Geometry: see drawing. Coordinates: mm, zero at the bounding-box minimum. Coordinates: 2 decimals unless noted, no trailing zeros. Write each loop counter-clockwise with the first axis right and the second up, starting at its lowest first coordinate (ties: lowest second). Pieces come first, ordered by that corner, then holes. Notation, with made-up numbers: (46.25, 41) - (94.25, 41) arc R15 cw to (94.25, 59) - close; hole circle Ø5 at (30.25, 79.25). An arc over 180 degrees is marked (long way). One line per question, with ' | ' between items. Start each with the question number.
1) Draft query along Z for the marked faces 1, 2 and 3. Return one class per face: released by +Z, released by -Z, zero draft, split by the parting line, or undercut.
2) Section query A-A on x = 10.5. Return loops of the section in (y, z).
3) Line query: line 1 (Z direction, x = 10.5, y = 4.6); line 2 (X direction, y = 1.45, z = 10.5). Output: solid intervals per line, ascending.
4) Section query C-C on y = 2.35. Return loops of the section in (x, z).
5) Section query B-B on z = 10.5. Return loops of the section in (x, y).
6) First-contact query: P1, Ø1, axis at x = 7.5, y = 4, coming from the +Z side; P2, Ø1.5, axis at x = 11, z = 18.5, coming from the +Y side. Flat tips, straight axial feed; report the tip coordinate or a pass-through.
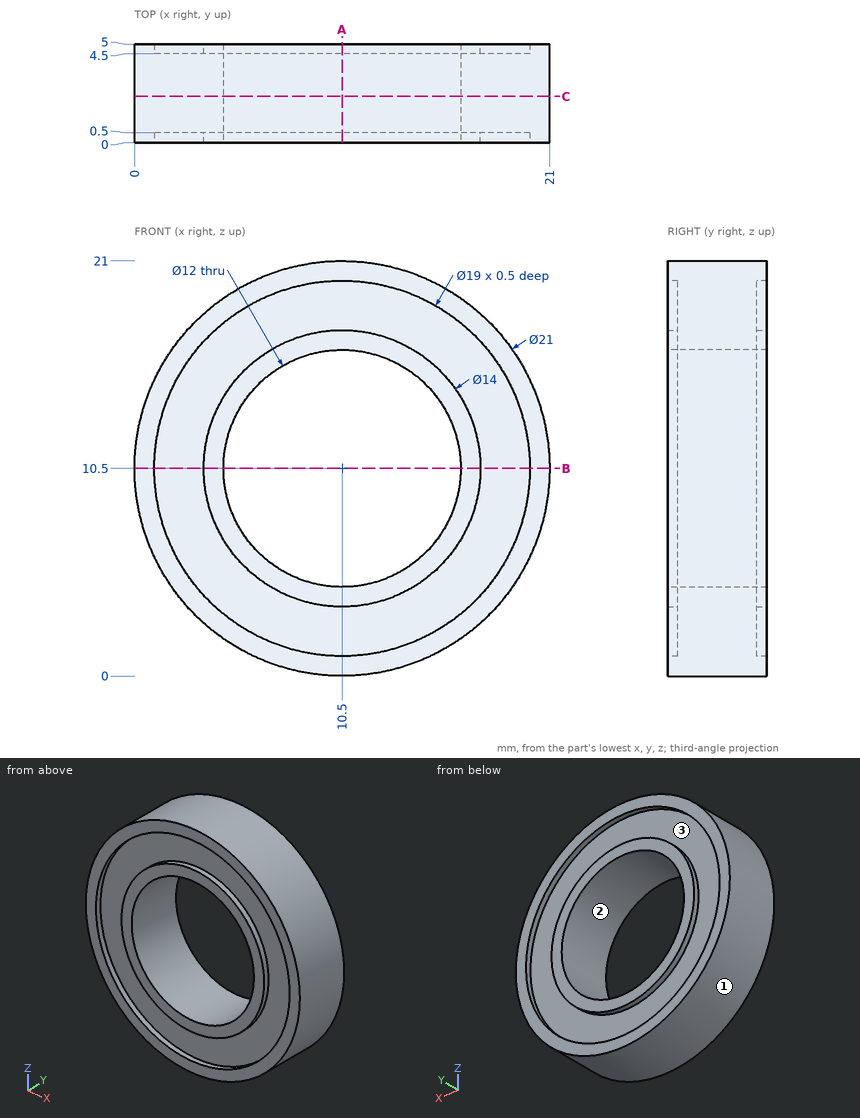
Answer key:
1) face 1: split by the parting line | face 2: undercut | face 3: undercut
2) outline: (0, 0) - (5, 0) - (5, 1) - (4.5, 1) - (4.5, 3.5) - (5, 3.5) - (5, 4.5) - (0, 4.5) - (0, 3.5) - (0.5, 3.5) - (0.5, 1) - (0, 1) - close; (0, 16.5) - (5, 16.5) - (5, 17.5) - (4.5, 17.5) - (4.5, 20) - (5, 20) - (5, 21) - (0, 21) - (0, 20) - (0.5, 20) - (0.5, 17.5) - (0, 17.5) - close
3) line 1: 0 to 1, 3.5 to 4.5, 16.5 to 17.5, 20 to 21 | line 2: 0 to 4.5, 16.5 to 21
4) outline: circle Ø21 at (10.5, 10.5); hole circle Ø12 at (10.5, 10.5)
5) outline: (0, 0) - (1, 0) - (1, 0.5) - (3.5, 0.5) - (3.5, 0) - (4.5, 0) - (4.5, 5) - (3.5, 5) - (3.5, 4.5) - (1, 4.5) - (1, 5) - (0, 5) - close; (16.5, 0) - (17.5, 0) - (17.5, 0.5) - (20, 0.5) - (20, 0) - (21, 0) - (21, 5) - (20, 5) - (20, 4.5) - (17.5, 4.5) - (17.5, 5) - (16.5, 5) - close
6) P1: z = 20.7 | P2: y = 4.5
